```python
from build123d import *

# Parameters (mm, degrees)
CROQUIS2_W              = 450
CROQUIS2_H              = 90
SALIENTE_EXTRUIR1_DEPTH = 10
CROQUIS6_R              = 18
CROQUIS6_R_2            = 2
CORTAR_EXTRUIR1_DEPTH   = 460.020696701
CHAFL_N5_SIZE           = 0.5
CROQUIS10_R             = 3.5
CROQUIS10_R_2           = 4.234641279
CROQUIS10_R_3           = 10
CORTAR_EXTRUIR3_DEPTH   = 460.020696701
CHAFL_N6_SIZE           = 0.5


with BuildPart() as part:
    # Croquis2 → Saliente-Extruir1 (new body)
    with BuildSketch(Plane.XY):
        with Locations((225, 45)):
            Rectangle(CROQUIS2_W, CROQUIS2_H)
    extrude(amount=SALIENTE_EXTRUIR1_DEPTH)

    # Croquis6 → Cortar-Extruir1 (cut, through all)
    with BuildSketch(Plane.XY.offset(10)):
        with Locations((225, 58)):
            Circle(CROQUIS6_R)
        with Locations((210.140026495, 72.838503544)):
            Circle(CROQUIS6_R_2)
        with Locations((239.838503544, 72.859973505)):
            Circle(CROQUIS6_R_2)
        with Locations((239.859973505, 43.161496456)):
            Circle(CROQUIS6_R_2)
        with Locations((210.161496456, 43.140026495)):
            Circle(CROQUIS6_R_2)
    extrude(amount=-CORTAR_EXTRUIR1_DEPTH, mode=Mode.SUBTRACT)

    # Chaflán5
    chafl_n5_edges = [part.edges().sort_by_distance(p)[0] for p in [
        (207, 58, 0),
        (207, 58, 10),
        (208.140026495, 72.838503544, 0),
        (208.140026495, 72.838503544, 10),
        (237.838503544, 72.859973505, 0),
        (237.838503544, 72.859973505, 10),
        (237.859973505, 43.161496456, 0),
        (237.859973505, 43.161496456, 10),
        (208.161496456, 43.140026495, 0),
        (208.161496456, 43.140026495, 10),
    ]]
    chamfer(chafl_n5_edges, length=CHAFL_N5_SIZE - 0.0001)  # a hair under: the kernel refuses the full size

    # Croquis10 → Cortar-Extruir3 (cut, through all)
    with BuildSketch(Plane.XY.offset(10)):
        with Locations((26, 50)):
            Circle(CROQUIS10_R)
        with Locations((74, 50)):
            Circle(CROQUIS10_R_2)
        with Locations(Location((376, 50, 0), (0, 0, 180))):
            Circle(CROQUIS10_R_2)
        with Locations(Location((400, 50, 0), (0, 0, 180))):
            Circle(CROQUIS10_R_3)
        with Locations((50, 50)):
            Circle(CROQUIS10_R_3)
        with Locations(Location((424, 50, 0), (0, 0, 180))):
            Circle(CROQUIS10_R)
    extrude(amount=-CORTAR_EXTRUIR3_DEPTH, mode=Mode.SUBTRACT)

    # Chaflán6
    chafl_n6_edges = [part.edges().sort_by_distance(p)[0] for p in [
        (427.5, 50, 0),
        (427.5, 50, 10),
        (22.5, 50, 0),
        (22.5, 50, 10),
        (69.765358721, 50, 0),
        (69.765358721, 50, 10),
        (380.234641279, 50, 0),
        (380.234641279, 50, 10),
        (410, 50, 0),
        (410, 50, 10),
        (40, 50, 0),
        (40, 50, 10),
    ]]
    chamfer(chafl_n6_edges, length=CHAFL_N6_SIZE)


solid = part.part
```
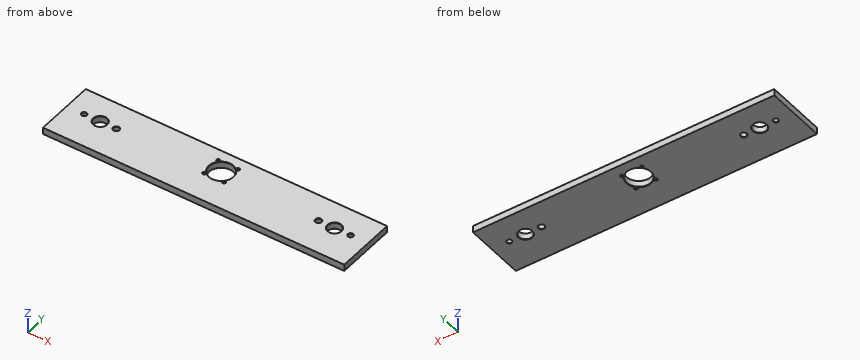
The listing builds one solid part. Answer for the finished solid, in the listing's coordinates (mm). Coordinates: 2 decimals unless noted, no trailing zeros. Write each loop counter-clockwise with the first axis right and the second up, starting at its lowest first coordinate (ties: lowest second). Pieces come first, ordered by that corner, then holes. Notation, with made-up numbers: (-31, -37) - (8, -37) arc R30 ccw to (8, -8) - close; hole circle Ø10 at (40, 25.5). An arc over 180 degrees is marked (long way). Return JSON: item names as keys, results as strings. Group by question number.
Q1. The part is cut by section B-B on z = 3.75. State how many separate pieces and enclosed holes the cut face has, and give its area (3 significant figures).
Q2. Flat-ended cylindrical pins translate along their axes: pin 1 Ø6.5 at (x, y) = (210.14, 72.84) entering from -Z; pin 2 Ø3.5 at (x, y) = (239.86, 43.16) entering from -Z; pin 3 Ø4.5 at (x, y) = (210.16, 43.14) entering from +Z. Find the tip coordinate at first contact, or state that the pin passes through.
Q3. The part is cut by section A-A on x = 74. Write down the section's boundary in (y, z).
Q4. The part is cut by section C-C on x = 400. Write down the section's boundary in (y, z), and give its area (4 significant figures).
Q5. Find the intervals of material crossed by line 1 along Y through (x, z) = (376, 5.25); line 2 along Z through (x, y) = (378.5, 46.5); line 3 along X through (y, z) = (61, 2.25), in increasing order. Write a range as [from, to].
Evaluation:
{
 "1": {"separate pieces": "1", "enclosed holes": "11", "area": "38,600 mm2"},
 "2": {"pin 1": "stops at z = 0", "pin 2": "passes through", "pin 3": "stops at z = 9.75"},
 "3": {"outline": "(0, 0) - (45.27, 0) - (45.77, 0.5) - (45.77, 9.5) - (45.27, 10) - (0, 10) - close; (54.23, 0.5) - (54.73, 0) - (90, 0) - (90, 10) - (54.73, 10) - (54.23, 9.5) - close"},
 "4": {"outline": "(0, 0) - (39.5, 0) - (40, 0.5) - (40, 9.5) - (39.5, 10) - (0, 10) - close; (60, 0.5) - (60.5, 0) - (90, 0) - (90, 10) - (60.5, 10) - (60, 9.5) - close", "area": "699.5 mm2"},
 "5": {"line 1": "y = [0, 45.77], [54.23, 90]", "line 2": "z = [0.43, 9.57]", "line 3": "x = [0, 207.25], [242.75, 450]"}
}
